For this review, take the finished solid that the model builds, in its own axes (mm). A direction names the side the tool comes from. Give positions to 0.01 mm unless a question says otherwise; leave off trailing zeros.
from build123d import *

# Parameters (mm, degrees)
BOSS_EXTRUDE2_DEPTH = 5.08
BOSS_EXTRUDE2_TAPER = 45
CUT_EXTRUDE1_DEPTH  = 28.788825452
CIRPATTERN1_COUNT   = 6
CUT_EXTRUDE2_DEPTH  = 4.572
CUT_EXTRUDE2_DRAFT  = -50
BOSS_EXTRUDE3_DEPTH = 1.5875


with BuildPart() as part:
    # Sketch2 → Boss-Extrude2 (new body)
    with BuildSketch(Plane(origin=(0, 0, 0), x_dir=(1, 0, 0), z_dir=(0, 1, 0))):
        Polygon((-11.156454307, -11.156454307), (-4.083545693, -15.24), (4.083545693, -15.24), (11.156454307, -11.156454307), (15.24, -4.083545693), (15.24, 4.083545693), (11.156454307, 11.156454307), (4.083545693, 15.24), (-4.083545693, 15.24), (-11.156454307, 11.156454307), (-15.24, 4.083545693), (-15.24, -4.083545693), align=None)
    extrude(amount=BOSS_EXTRUDE2_DEPTH, taper=BOSS_EXTRUDE2_TAPER)

    # Sketch3 → Cut-Extrude1 (cut, through all)
    with BuildSketch(Plane(origin=(-1.499582091, 7.605575605, 5.596516554), x_dir=(-0.9876151240341646, -0.12385705516936496, -0.09631093740460966), z_dir=(0.15684209814252395, -0.795471246716067, -0.5853426790336042))):
        Polygon((-4.296360621, -5.154612088), (6.000002448, -3.004781355), (2.5651928, -12.285691151), align=None)
    cut_extrude1 = extrude(amount=-CUT_EXTRUDE1_DEPTH, mode=Mode.SUBTRACT)

    # CirPattern1: Cut-Extrude1 ×6 about axis
    cirpattern1_axis = Axis((0, 0, 0), (0, 1, 0))
    for i in range(1, CIRPATTERN1_COUNT):
        add(cut_extrude1.rotate(cirpattern1_axis, i * 360 / CIRPATTERN1_COUNT), mode=Mode.SUBTRACT)


with BuildPart() as cut_extrude2_tool:
    # Sketch5 → Cut-Extrude2 (with draft: the straight prism first)
    with BuildSketch(Plane.XZ):
        Polygon((13.933401039, -3.877261622), (14.005310072, 3.608893457), (10.324507581, 10.12804845), (3.877261622, 13.933401039), (-3.608893457, 14.005310072), (-10.12804845, 10.324507581), (-13.933401039, 3.877261622), (-14.005310072, -3.608893457), (-10.324507581, -10.12804845), (-3.877261622, -13.933401039), (3.608893457, -14.005310072), (10.12804845, -10.324507581), align=None)
    extrude(amount=-CUT_EXTRUDE2_DEPTH)
    # Cut-Extrude2: the draft: its side faces are tilted about the plane it starts from
    cut_extrude2_sides = [cut_extrude2_tool.faces().sort_by_distance(p)[0] for p in [
        (13.969355555, 2.286, -0.134184083),
        (12.164908827, 2.286, 6.868470953),
        (7.100884602, 2.286, 12.030724744),
        (0.134184083, 2.286, 13.969355555),
        (-6.868470953, 2.286, 12.164908827),
        (-12.030724744, 2.286, 7.100884602),
        (-13.969355555, 2.286, 0.134184083),
        (-12.164908827, 2.286, -6.868470953),
        (-7.100884602, 2.286, -12.030724744),
        (-0.134184083, 2.286, -13.969355555),
        (6.868470953, 2.286, -12.164908827),
        (12.030724744, 2.286, -7.100884602),
    ]]
    draft(cut_extrude2_sides, Plane.XZ, CUT_EXTRUDE2_DRAFT)


with BuildPart() as part_1:
    add(part.part)

    # Cut-Extrude2: cut by cut_extrude2_tool
    add(cut_extrude2_tool.part, mode=Mode.SUBTRACT)

    # Sketch8 → Boss-Extrude3 (add)
    with BuildSketch(Plane.XZ):
        Polygon((-15.24, -4.083545693), (-11.156454307, -11.156454307), (-4.083545693, -15.24), (4.083545693, -15.24), (11.156454307, -11.156454307), (15.24, -4.083545693), (15.24, 4.083545693), (11.156454307, 11.156454307), (4.083545693, 15.24), (-4.083545693, 15.24), (-11.156454307, 11.156454307), (-15.24, 4.083545693), align=None)
        Polygon((-10.12804845, 10.324507581), (-13.933401039, 3.877261622), (-14.005310072, -3.608893457), (-10.324507581, -10.12804845), (-3.877261622, -13.933401039), (3.608893457, -14.005310072), (10.12804845, -10.324507581), (13.933401039, -3.877261622), (14.005310072, 3.608893457), (10.324507581, 10.12804845), (3.877261622, 13.933401039), (-3.608893457, 14.005310072), align=None, mode=Mode.SUBTRACT)
    extrude(amount=BOSS_EXTRUDE3_DEPTH)


solid = part_1.part
1) To check wall thickness, follow line 1 (Z direction, x = -7, y = 3.25); line 2 (X direction, y = 2.5, z = 1); line 3 (Z direction, x = 12.5, y = 0.25). State the ranges of each line that lie inside material, in increasing order.
Answer sheet:
line 1: z = -9.28 to -7.59, 7.64 to 9.8
line 2: x = -12.67 to -10.98, 11 to 12.74
line 3: z = -8.33 to -5.72, 5.67 to 8.33
2) Tool access review of faces 1 (the face through (-12, -0.78, 7.15)), 2 (the face through (-8.116, 3.606, -7.502)): name each direction out of +Z, -Z, +X, -X, +Y, -Y from which nothing blocks a thin tool from reaching the whole face with its end or side.
Answer sheet:
face 1: -Y
face 2: -Z, -X, +Y
3) Clearance check with flat-ended pins moving along their axes: pin 1 (4 mm diameter, centred on y = 2, z = 10.5, fed in from +X); pin 2 (1 mm diameter, centred on x = 0, z = -9, fed in from -Y); pin 3 (8.5 mm diameter, centred on x = 0.5, z = -3.5, fed in from -Y). State where each tip first meets the part, or that it passes through.
Answer sheet:
pin 1: stops at x = 11.81
pin 2: stops at y = 3.75
pin 3: stops at y = 4.57
